Geometry check sheet. Reference: the model listing, model coordinates, mm. Face numbers are marked on the shaded views. A direction names the side the tool comes from. Coordinates: 2 decimals unless noted, no trailing zeros. Order: outer loops, then holes, each group sorted by start corner. A loop starts at its lowest first (then second) coordinate and runs counter-clockwise, first axis right, second up. Notation, with made-up numbers: M -16.5,46 L -4.5,46 A3 cw -4.5,51 Z; hole C 79.25,3 d2. An arc over 180 degrees is marked long. One line per item, written item: value. Start each with the question number.
1) Sectioned sample at A-A, the plane x = 0.75. Enter the section's corners in (y, z) (3 decimals), then the cut area to 3 significant figures.
2) Thickness scan on L1, parallel to Y at x = 3.25, z = 4.25 (3 decimals); L2, parallel to X at y = -2.75, z = 9.25 (3 decimals); L3, parallel to Z at x = 4.6, y = -1. Record the ranges inside material, lowest first. Write a range as from..to.
3) Go/stop test with flat-tipped pins: P1, Ø2, axis at x = 4.5, z = 7.5, coming from the +Y side (3 decimals); P2, Ø0.6, axis at x = 1.5, y = 4, coming from the +Z side; P3, Ø1, axis at x = 1, z = 10, coming from the -Y side (3 decimals). Record where each tip stops, or that it passes through.
4) Sectioned sample at C-C, the plane y = 4. Enter the section's corners in (x, z), then the cut area to 3 significant figures.
5) Access from +Z, -Z, +X, -X, +Y, -Y to the whole of each face (thin tool, end or side, straight path). Record for the marked faces 1, 2 and 3.
6) Sectioned sample at B-B, the plane z = 10. Enter the section's corners in (x, y) (3 decimals), then the cut area to 3 significant figures.
7) Sectioned sample at D-D, the plane x = 4.75. Enter the section's corners in (y, z) (3 decimals).
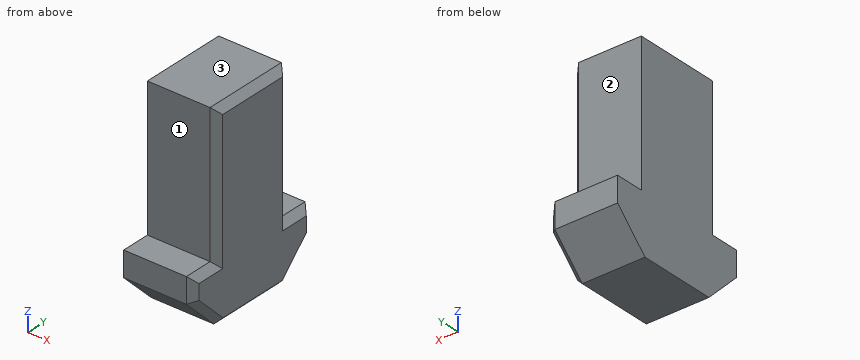
```python
from build123d import *

# Parameters (mm, degrees)
BOSS_EXTRUDE1_DEPTH = 5
CHAMFER1_SIZE       = 0.5


with BuildPart() as part:
    # Sketch2 → Boss-Extrude1 (new body)
    with BuildSketch(Plane(origin=(0, 0, 0), x_dir=(0, 0, -1), z_dir=(1, 0, 0))):
        Polygon((-4.2, 3.125), (-14.2, 3.125), (-14.2, -3.125), (-4.2, -3.125), (-4.2, -5.2), (-2.4, -5.2), (0, -2.8), (0, 2.8), (-2.4, 5.2), (-4.2, 5.2), align=None)
    extrude(amount=BOSS_EXTRUDE1_DEPTH)

    # Chamfer1
    chamfer1_edges = [part.edges().sort_by_distance(p)[0] for p in [
        (5, 0, 14.2),
        (5, -3.125, 9.2),
        (5, -4.1625, 4.2),
        (5, -5.2, 3.3),
        (5, -4, 1.2),
        (5, 0, 0),
        (5, 4, 1.2),
        (5, 5.2, 3.3),
        (5, 4.1625, 4.2),
        (5, 3.125, 9.2),
    ]]
    chamfer(chamfer1_edges, length=CHAMFER1_SIZE)


solid = part.part
```
Final values:
1. outline: M -5.2,2.4 L -2.8,0 L 2.8,0 L 5.2,2.4 L 5.2,4.2 L 3.125,4.2 L 3.125,14.2 L -3.125,14.2 L -3.125,4.2 L -5.2,4.2 Z
1. area: 100 mm^2
2. L1: y = -3.125..3.125
2. L2: x = 0..4.875
2. L3: z = 0.1..14.1
3. P1: stops at y = 3.125
3. P2: stops at z = 4.2
3. P3: stops at y = -3.125
4. outline: M 0,1.2 L 4.5,1.2 L 5,1.91 L 5,3.7 L 4.5,4.2 L 0,4.2 Z
4. area: 14.7 mm^2
5. face 1: +Z, +X, -X, -Y
5. face 2: +Z, +X, -X, +Y
5. face 3: +Z, +X, -X, +Y, -Y
6. outline: M 0,-3.125 L 4.5,-3.125 L 5,-2.625 L 5,2.625 L 4.5,3.125 L 0,3.125 Z
6. area: 31.0 mm^2
7. outline: M -4.95,2.504 L -2.696,0.25 L 2.696,0.25 L 4.95,2.504 L 4.95,3.95 L 2.875,3.95 L 2.875,13.95 L -2.875,13.95 L -2.875,3.95 L -4.95,3.95 Z
